```python
from build123d import *

# Parameters (mm, degrees)
SKETCH_W             = 100
SKETCH_H             = 100
SKETCH_W_2           = 30
SKETCH_H_2           = 30
PAD_DEPTH            = 200
BODY_PLACEMENT_ANGLE = 90


with BuildPart() as part:
    # Sketch → Pad (new body)
    with BuildSketch(Plane.XY):
        Rectangle(SKETCH_W, SKETCH_H)
        with Locations((-25.244661, 25.084817)):
            Rectangle(SKETCH_W_2, SKETCH_H_2, mode=Mode.SUBTRACT)
        with Locations((-25.244661, -25.084817)):
            Rectangle(SKETCH_W_2, SKETCH_H_2, mode=Mode.SUBTRACT)
        with Locations((25.244661, 25.084817)):
            Rectangle(SKETCH_W_2, SKETCH_H_2, mode=Mode.SUBTRACT)
        with Locations((25.244661, -25.084817)):
            Rectangle(SKETCH_W_2, SKETCH_H_2, mode=Mode.SUBTRACT)
    extrude(amount=PAD_DEPTH)


with BuildPart() as part_1:
    # Body placement: moved
    add(part.part.rotate(Axis((0, 0, 0), (0, 1, 0)), BODY_PLACEMENT_ANGLE))


solid = part_1.part
```
Source: CAD feature listing. Evaluate the final solid. Frame: model axes, mm. A direction names the side the tool comes from. Coordinates: 2 decimals unless noted, no trailing zeros. Write each loop counter-clockwise with the first axis right and the second up, starting at its lowest first coordinate (ties: lowest second). Pieces come first, ordered by that corner, then holes. Notation, with made-up numbers: M 30.5,-25.5 L 79.5,-25.5 A11 ccw 79.5,-9.5 Z; hole C 69,-4.5 d1. An arc over 180 degrees is marked long. Answer as a JSON object with one key per item and string values.
1. Cut plane C-C on z = 20. Output: boundary loops of the cut face in (x, y).
Evaluation:
{"outline": "M 0,-50 L 200,-50 L 200,-40.08 L 0,-40.08 Z; M 0,-10.08 L 200,-10.08 L 200,10.08 L 0,10.08 Z; M 0,40.08 L 200,40.08 L 200,50 L 0,50 Z"}
2. Ray query, L1, parallel to Z at x = 119.5, y = 23; L2, parallel to Y at x = 47.5, z = 23. Return the intervals inside material, ascending.
Evaluation:
{"L1": "-50 to -40.24, -10.24 to 10.24, 40.24 to 50", "L2": "-50 to -40.08, -10.08 to 10.08, 40.08 to 50"}
3. Cut plane B-B on y = 17. Output: boundary loops of the cut face in (x, z).
Evaluation:
{"outline": "M 0,-50 L 200,-50 L 200,-40.24 L 0,-40.24 Z; M 0,-10.24 L 200,-10.24 L 200,10.24 L 0,10.24 Z; M 0,40.24 L 200,40.24 L 200,50 L 0,50 Z"}
4. Draft query along Y for faces 3 (the flat face through (99, -50, 1)), 4 (the flat face through (99, 10.085, -25)), 5 (the flat face through (99, -1, -50)). Return one class per face: released by +Y, released by -Y, zero draft, split by the parting line, or undercut.
Evaluation:
{"face 3": "released by -Y", "face 4": "undercut", "face 5": "zero draft"}
5. Access query for faces 1 (the flat face through (99, -25, -40.245)), 2 (the flat face through (200, 1, 1)). Directions: +Z, -Z, +X, -X, +Y, -Y. A direction counts if a zero-diameter tool reaches every point of the face in a straight line with its end or side. Return the directions, or none.
Evaluation:
{"face 1": "+X, -X", "face 2": "+Z, -Z, +X, +Y, -Y"}
6. Cut plane A-A on x = 104. Output: boundary loops of the cut face in (y, z), plus the area to 3 significant figures.
Evaluation:
{"outline": "M -50,-50 L 50,-50 L 50,50 L -50,50 Z; hole M -40.08,-40.24 L -10.08,-40.24 L -10.08,-10.24 L -40.08,-10.24 Z; hole M -40.08,10.24 L -10.08,10.24 L -10.08,40.24 L -40.08,40.24 Z; hole M 10.08,-40.24 L 40.08,-40.24 L 40.08,-10.24 L 10.08,-10.24 Z; hole M 10.08,10.24 L 40.08,10.24 L 40.08,40.24 L 10.08,40.24 Z", "area": "6,400 mm^2"}
